Model file for the job. Use its own axes, mm. Face numbers are marked on the shaded views. A direction names the side the tool comes from. Round coordinates to 2 decimals unless told otherwise and drop trailing zeros. Order: outer loops, then holes, each group sorted by start corner. A loop starts at its lowest first (then second) coordinate and runs counter-clockwise, first axis right, second up. Notation, with made-up numbers: (74.5, 57.25) - (132.5, 57.25) arc R17 cw to (132.5, 85.25) - close; hole circle Ø4 at (37, 66.25). An arc over 180 degrees is marked (long way). Write item = value, one per line. Start each with the question number.
from build123d import *

# Parameters (mm, degrees)
SKETCH1_W           = 164
SKETCH1_H           = 84
BOSS_EXTRUDE1_DEPTH = 33
SHELL1_T            = -2
SKETCH3_W           = 142
SKETCH3_H           = 62
CUT_EXTRUDE1_DEPTH  = 2
SKETCH4_R           = 3
BOSS_EXTRUDE2_DEPTH = 2
SKETCH5_R           = 1.5
BOSS_EXTRUDE3_DEPTH = 4
SKETCH6_R           = 3
BOSS_EXTRUDE4_DEPTH = 2
SKETCH7_R           = 1.5
BOSS_EXTRUDE5_DEPTH = 4
SKETCH8_W           = 64
SKETCH8_H           = 12
CUT_EXTRUDE2_DEPTH  = 188.192414376
SKETCH9_W           = 144
SKETCH9_H           = 12
CUT_EXTRUDE3_DEPTH  = 188.192414376


with BuildPart() as part:
    # Sketch1 → Boss-Extrude1 (new body)
    with BuildSketch(Plane(origin=(0, 0, 0), x_dir=(1, 0, 0), z_dir=(0, 1, 0))):
        with Locations((82, 42)):
            Rectangle(SKETCH1_W, SKETCH1_H)
    extrude(amount=BOSS_EXTRUDE1_DEPTH)

    # Shell1
    shell1_openings = [part.faces().sort_by_distance(p)[0] for p in [
        (82, 33, -42),
    ]]
    offset(amount=SHELL1_T, openings=shell1_openings, kind=Kind.INTERSECTION)

    # Sketch3 → Cut-Extrude1 (cut)
    with BuildSketch(Plane(origin=(0, 2, 0), x_dir=(1, 0, 0), z_dir=(0, 1, 0))):
        with Locations((82, 42)):
            Rectangle(SKETCH3_W, SKETCH3_H)
    extrude(amount=-CUT_EXTRUDE1_DEPTH, mode=Mode.SUBTRACT)

    # Sketch4 → Boss-Extrude2 (add)
    with BuildSketch(Plane(origin=(0, 2, 0), x_dir=(1, 0, 0), z_dir=(0, 1, 0))):
        with Locations(Location((157, 76, 0), (0, 0, 90))):
            Circle(SKETCH4_R)
        with Locations(Location((89, 76, 0), (0, 0, 270))):
            Circle(SKETCH4_R)
        with Locations(Location((89, 8, 0), (0, 0, 90))):
            Circle(SKETCH4_R)
        with Locations(Location((157, 8, 0), (0, 0, 90))):
            Circle(SKETCH4_R)
    extrude(amount=BOSS_EXTRUDE2_DEPTH)

    # Sketch5 → Boss-Extrude3 (add)
    with BuildSketch(Plane(origin=(0, 4, 0), x_dir=(1, 0, 0), z_dir=(0, 1, 0))):
        with Locations(Location((89, 76, 0), (0, 0, 270))):
            Circle(SKETCH5_R)
        with Locations(Location((157, 76, 0), (0, 0, 270))):
            Circle(SKETCH5_R)
        with Locations(Location((89, 8, 0), (0, 0, 270))):
            Circle(SKETCH5_R)
        with Locations(Location((157, 8, 0), (0, 0, 270))):
            Circle(SKETCH5_R)
    extrude(amount=BOSS_EXTRUDE3_DEPTH)

    # Sketch6 → Boss-Extrude4 (add)
    with BuildSketch(Plane(origin=(0, 2, 0), x_dir=(1, 0, 0), z_dir=(0, 1, 0))):
        with Locations(Location((7, 76, 0), (0, 0, 90))):
            Circle(SKETCH6_R)
        with Locations(Location((7, 8, 0), (0, 0, 90))):
            Circle(SKETCH6_R)
        with Locations(Location((63, 8, 0), (0, 0, 90))):
            Circle(SKETCH6_R)
    extrude(amount=BOSS_EXTRUDE4_DEPTH)

    # Sketch7 → Boss-Extrude5 (add)
    with BuildSketch(Plane(origin=(0, 4, 0), x_dir=(1, 0, 0), z_dir=(0, 1, 0))):
        with Locations(Location((7, 76, 0), (0, 0, 270))):
            Circle(SKETCH7_R)
        with Locations(Location((7, 8, 0), (0, 0, 270))):
            Circle(SKETCH7_R)
        with Locations(Location((63, 8, 0), (0, 0, 270))):
            Circle(SKETCH7_R)
    extrude(amount=BOSS_EXTRUDE5_DEPTH)

    # Sketch8 → Cut-Extrude2 (cut, through all)
    with BuildSketch(Plane.ZY):
        with Locations((-42, 22)):
            Rectangle(SKETCH8_W, SKETCH8_H)
    extrude(amount=-CUT_EXTRUDE2_DEPTH, mode=Mode.SUBTRACT)

    # Sketch9 → Cut-Extrude3 (cut, through all)
    with BuildSketch(Plane.XY):
        with Locations((82, 22)):
            Rectangle(SKETCH9_W, SKETCH9_H)
    extrude(amount=-CUT_EXTRUDE3_DEPTH, mode=Mode.SUBTRACT)


solid = part.part
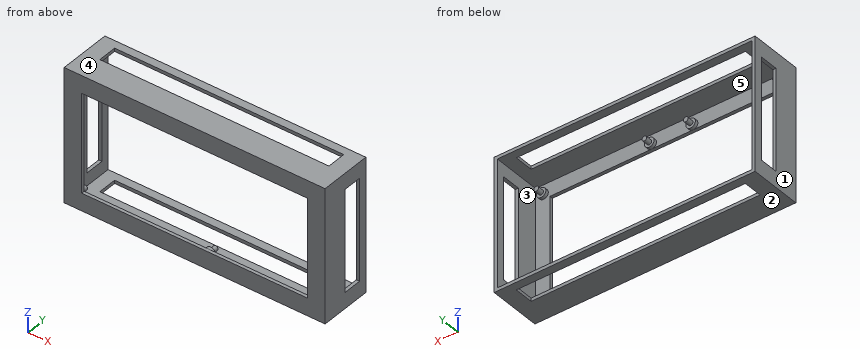
Item 1: Saw through at B-B, the plane y = 10. Give the cut face in (x, z), then the cut area to 3 significant figures.
Item 2: Which spindle directions (+Z, -Z, +X, -X, +Y, -Y) get a long thin tool onto all of the face, cutting with end or side? Do the marked faces 4 and 5. Say none if no direction does.
Item 3: Saw through at C-C, the plane z = -24.5. Give the cut face in (x, y).
Item 4: Drop a flat-ended pin along its axis: pin 1 (1.5 mm diameter, centred on x = 89.5, z = -76.5, fed in from +Y). Give the stop position or say it passes through.
Item 5: Mould opens along Z. For the marked faces 1, 2 and 3 say: +Z half, -Z half, draft (parallel to the pull), parting line (faces both ways), or undercut.
Item 6: Saw through at A-A, the plane x = 129. Give the cut face in (y, z).
Item 7: Probe L1, parallel to Z at x = 121, y = 3; L2, parallel to Z at x = 89, y = 5.5; L3, parallel to X at y = 4.5, z = -57. List the from-to ranges inside material, lowest first.
Item 8: Saw through at D-D, the plane y = 20. Give the cut face in (x, z), then the cut area to 3 significant figures.
Check sheet entries:
q1.outline = (0, -84) - (164, -84) - (164, 0) - (0, 0) - close; hole (2, -82) - (162, -82) - (162, -2) - (2, -2) - close
q1.area = 976 mm2
q2.face_4 = +Z, +X, -X, +Y, -Y
q2.face_5 = +Y
q3.outline = (0, 0) - (11, 0) - (11, 2) - (2, 2) - (2, 16) - (0, 16) - close; (0, 28) - (2, 28) - (2, 33) - (0, 33) - close; (153, 0) - (164, 0) - (164, 16) - (162, 16) - (162, 2) - (153, 2) - close; (162, 28) - (164, 28) - (164, 33) - (162, 33) - close
q4.pin_1 = 8
q5.face_1 = draft
q5.face_2 = -Z half
q5.face_3 = undercut
q6.outline = (0, -84) - (16, -84) - (16, -82) - (2, -82) - (2, -73) - (0, -73) - close; (0, -11) - (2, -11) - (2, -2) - (16, -2) - (16, 0) - (0, 0) - close; (28, -84) - (33, -84) - (33, -82) - (28, -82) - close; (28, -2) - (33, -2) - (33, 0) - (28, 0) - close
q7.L1 = -84 to -82, -2 to 0
q7.L2 = -84 to -82, -77.5 to -74.5, -9.5 to -6.5, -2 to 0
q7.L3 = 0 to 2, 162 to 164
q8.outline = (0, -84) - (10, -84) - (10, -82) - (2, -82) - (2, -74) - (0, -74) - close; (0, -10) - (2, -10) - (2, -2) - (10, -2) - (10, 0) - (0, 0) - close; (154, -84) - (164, -84) - (164, -74) - (162, -74) - (162, -82) - (154, -82) - close; (154, -2) - (162, -2) - (162, -10) - (164, -10) - (164, 0) - (154, 0) - close
q8.area = 144 mm2
